Geometry check sheet. Reference: the model listing, model coordinates, mm. A direction names the side the tool comes from. Give positions to 0.01 mm unless a question says otherwise; leave off trailing zeros. Write each loop counter-clockwise with the first axis right and the second up, starting at its lowest first coordinate (ties: lowest second). Pieces come first, ordered by that corner, then holes. Notation, with made-up numbers: M 42,84.5 L 70,84.5 A24 cw 70,104.5 Z; hole C 0.5,9.5 d3. An arc over 180 degrees is marked long. One line per item, written item: value. Start each with the question number.
1. Release check for a two-part mould opening along Z. For faces 6 (the face through (64, 4, 2)), 7 (the face through (9.493, 68.474, 30.981)), 8 (the face through (61.86, 45.9, 19.74)) record: pulls with the +Z half, pulls with the -Z half, needs draft (parallel to the pull), parting line crosses it, or undercut.
2. Tool access check on faces 1 (the face through (-4, 82, 3)), 2 (the face through (67.43, 87.4, 19.27)), 3 (the face through (62.9, 5.1, 37)), 4 (the face through (68, 43, 19)), 5 (the face through (0, 26, 19)). Record the directions out of +Z, -Z, +X, -X, +Y, -Y that give a thin tool (end or side, any length) a straight path to the whole face; none if there is none.
3. Cross-section at B-B on x = 50. Record the cut outline in (y, z), then the cut area to 3 significant figures.
4. Cross-section at D-D on y = 10.5. Record the cut outline in (x, z), then the cut area to 3 significant figures.
5. Gauge pin test, flat ends, axial feed: pin 1 (3 mm diameter, centred on x = 64, y = 4.5, fed in from +Z); pin 2 (19 mm diameter, centred on y = 15, z = 13.5, fed in from -X); pin 3 (1.5 mm diameter, centred on y = 75, z = 13, fed in from -X). Record the tip position at first contact, or that the pin passes through.
6. Cross-section at A-A on y = 70. Count the separate pieces of the cut face and the enclosed holes in it, then the cut area to 3 significant figures.
7. Scan lines: line 1 (Z direction, x = 9.4, y = 70); line 2 (Y direction, x = 2.5, z = 17); line 3 (Y direction, x = 4, z = 22). Record each from-to range of solid material in increasing order.
from build123d import *

# Parameters (mm, degrees)
EXTRUDE_1_DEPTH     = 38
SHELL_1_T           = -2
SKETCH_9_W          = 20
SKETCH_9_H          = 34.8
EXTRUDE_3_DEPTH     = 6
SKETCH_9_3_W        = 20
SKETCH_9_3_H        = 1.2
EXTRUDE_4_DEPTH     = 38
FILLET_1_R          = 2
FILLET_2_R          = 4
FILLET_4_R          = 2
SKETCH_3_W          = 6
SKETCH_3_H          = 6
SKETCH_3_R          = 1.4
EXTRUDE_2_DEPTH     = 35
FILLET_3_R          = 3
SKETCH_2_R          = 3.75
SKETCH_2_R_2        = 1.6
CUT_EXTRUDE_1_DEPTH = 30
CHAMFER_1_SIZE      = 1
CUT_EXTRUDE_START   = -2
SKETCH_2_3_R        = 12.5
CUT_EXTRUDE_2_DEPTH = 5
CUT_EXTRUDE_START_2 = 1.2
CUT_EXTRUDE_4_DEPTH = 10
SKETCH_10_R         = 1.4
CUT_EXTRUDE_5_DEPTH = 8
SKETCH_11_W         = 56
SKETCH_11_H         = 6
SKETCH_11_R         = 1.4
EXTRUDE_5_DEPTH     = 6
SKETCH_11_2_R       = 1.4
CUT_EXTRUDE_6_DEPTH = 6


with BuildPart() as part:
    # 草图1 → 凸台-拉伸1 (new body)
    with BuildSketch(Plane.XY):
        Polygon((0, 0), (68, 0), (68, 88), (8, 88), (8, 52), (0, 52), align=None)
    extrude(amount=EXTRUDE_1_DEPTH)

    # 抽壳1
    shell_1_openings = [part.faces().sort_by_distance(p)[0] for p in [
        (35.516853933, 42.685393258, 38),
    ]]
    offset(amount=SHELL_1_T, openings=shell_1_openings, kind=Kind.INTERSECTION)

    # 草图9 → 凸台-拉伸3 (add)
    with BuildSketch(Plane.XY):
        with Locations((-2, 69.4)):
            Rectangle(SKETCH_9_W, SKETCH_9_H)
    extrude(amount=EXTRUDE_3_DEPTH)

    # 草图9<3> → 凸台-拉伸4 (add)
    with BuildSketch(Plane.XY):
        with Locations((-2, 87.4)):
            Rectangle(SKETCH_9_3_W, SKETCH_9_3_H)
    extrude(amount=EXTRUDE_4_DEPTH)

    # 圆角1
    fillet_1_edges = [part.edges().sort_by_distance(p)[0] for p in [
        (0, 0, 19),
        (8, 52, 22),
        (68, 88, 19),
        (68, 0, 19),
        (0, 52, 3),
        (8, 86.8, 22),
    ]]
    fillet(fillet_1_edges, radius=FILLET_1_R)

    # 圆角2
    fillet_2_edges = [part.edges().sort_by_distance(p)[0] for p in [
        (10, 50, 20),
        (-12, 52, 3),
    ]]
    fillet(fillet_2_edges, radius=FILLET_2_R)

    # 圆角4
    fillet_4_edges = [part.edges().sort_by_distance(p)[0] for p in [
        (0, 52, 22),
    ]]
    fillet(fillet_4_edges, radius=FILLET_4_R)

    # 草图3 → 凸台-拉伸2 (add)
    # profile 1 of 6: a face of its own
    with BuildSketch(Plane.XY.offset(2)):
        with Locations((64, 84)):
            Rectangle(SKETCH_3_W, SKETCH_3_H)
        with Locations((64, 84)):
            Circle(SKETCH_3_R, mode=Mode.SUBTRACT)
    # profile 2 of 6: a face of its own
    with BuildSketch(Plane.XY.offset(2)):
        with Locations((12, 84)):
            Rectangle(SKETCH_3_W, SKETCH_3_H)
        with Locations((12, 84)):
            Circle(SKETCH_3_R, mode=Mode.SUBTRACT)
    # profile 3 of 6: a face of its own
    with BuildSketch(Plane.XY.offset(2)):
        with Locations((64, 4)):
            Rectangle(SKETCH_3_W, SKETCH_3_H)
        with Locations((64, 4)):
            Circle(SKETCH_3_R, mode=Mode.SUBTRACT)
    # profile 4 of 6: a face of its own
    with BuildSketch(Plane.XY.offset(2)):
        with Locations((4, 48)):
            Rectangle(SKETCH_3_W, SKETCH_3_H)
        with Locations((4, 48)):
            Circle(SKETCH_3_R, mode=Mode.SUBTRACT)
    # profile 5 of 6: a face of its own
    with BuildSketch(Plane.XY.offset(2)):
        with Locations((4, 4)):
            Rectangle(SKETCH_3_W, SKETCH_3_H)
        with Locations((4, 4)):
            Circle(SKETCH_3_R, mode=Mode.SUBTRACT)
    # profile 6 of 6: a face of its own
    with BuildSketch(Plane.XY.offset(2)):
        with Locations((64, 48)):
            Rectangle(SKETCH_3_W, SKETCH_3_H)
        with Locations((64, 48)):
            Circle(SKETCH_3_R, mode=Mode.SUBTRACT)
    extrude(amount=EXTRUDE_2_DEPTH)

    # 圆角3
    fillet_3_edges = [part.edges().sort_by_distance(p)[0] for p in [
        (15, 81, 19.5),
        (61, 81, 19.5),
        (61, 7, 19.5),
        (7, 45, 19.5),
        (7, 7, 19.5),
        (61, 45, 19.5),
        (61, 51, 19.5),
    ]]
    fillet(fillet_3_edges, radius=FILLET_3_R - 0.0001)  # a hair under: the kernel refuses the full size

    # 草图2 → 切除-拉伸1 (cut)
    with BuildSketch(Plane.ZY.offset(-8)):
        with Locations(Location((22, 70, 0), (0, 0, 270))):
            Circle(SKETCH_2_R)
        with Locations(Location((30.5, 70, 0), (0, 0, 270))):
            Circle(SKETCH_2_R_2)
        with Locations(Location((13.5, 70, 0), (0, 0, 270))):
            Circle(SKETCH_2_R_2)
    extrude(amount=-CUT_EXTRUDE_1_DEPTH, mode=Mode.SUBTRACT)

    # 倒角1
    chamfer_1_edges = [part.edges().sort_by_distance(p)[0] for p in [
        (8, 71.6, 13.5),
        (8, 71.6, 30.5),
    ]]
    chamfer(chamfer_1_edges, length=CHAMFER_1_SIZE)

    # 草图2<3> → 切除-拉伸2 (cut)
    with BuildSketch(Plane.ZY.offset(-8).offset(CUT_EXTRUDE_START)):
        with Locations((22, 70)):
            Circle(SKETCH_2_3_R)
    extrude(amount=-CUT_EXTRUDE_2_DEPTH, mode=Mode.SUBTRACT)

    # 草图1<3> → 切除-拉伸4 (cut)
    with BuildSketch(Plane.XY.offset(CUT_EXTRUDE_START_2)):
        Polygon((8, 44), (8, 8), (60, 8), (60, 80), (16, 80), (16, 44), align=None)
    extrude(amount=CUT_EXTRUDE_4_DEPTH, mode=Mode.SUBTRACT)

    # 草图10 → 切除-拉伸5 (cut)
    with BuildSketch(Plane.ZY.offset(12)):
        with Locations(Location((3, 82, 0), (0, 0, 270))):
            Circle(SKETCH_10_R)
        with Locations(Location((3, 62, 0), (0, 0, 270))):
            Circle(SKETCH_10_R)
    extrude(amount=-CUT_EXTRUDE_5_DEPTH, mode=Mode.SUBTRACT)

    # 草图11 → 凸台-拉伸5 (add)
    with BuildSketch(Plane.XZ):
        with Locations((34, 3)):
            Rectangle(SKETCH_11_W, SKETCH_11_H)
        with Locations((10, 3)):
            Circle(SKETCH_11_R, mode=Mode.SUBTRACT)
        with Locations((34, 3)):
            Circle(SKETCH_11_R, mode=Mode.SUBTRACT)
        with Locations((58, 3)):
            Circle(SKETCH_11_R, mode=Mode.SUBTRACT)
    extrude(amount=-EXTRUDE_5_DEPTH)

    # 草图11<2> → 切除-拉伸6 (cut)
    with BuildSketch(Plane.XZ):
        with Locations(Location((10, 3, 0), (0, 0, 270))):
            Circle(SKETCH_11_2_R)
        with Locations(Location((58, 3, 0), (0, 0, 270))):
            Circle(SKETCH_11_2_R)
        with Locations(Location((34, 3, 0), (0, 0, 270))):
            Circle(SKETCH_11_2_R)
    extrude(amount=-CUT_EXTRUDE_6_DEPTH, mode=Mode.SUBTRACT)


solid = part.part
Report:
1. face 6: pulls with the +Z half
1. face 7: undercut
1. face 8: needs draft
2. face 1: -X
2. face 2: +Z, -Z, +X, +Y
2. face 3: +Z
2. face 4: +Z, -Z, +X, +Y, -Y
2. face 5: +Z, -Z, -X, -Y
3. outline: M 0,0 L 88,0 L 88,38 L 86,38 L 86,2 L 80,2 L 80,1.2 L 8,1.2 L 8,2 L 6,2 L 6,6 L 2,6 L 2,38 L 0,38 Z
3. area: 278 mm^2
4. outline: M 0,0 L 68,0 L 68,38 L 66,38 L 66,2 L 60,2 L 60,1.2 L 8,1.2 L 8,2 L 2,2 L 2,38 L 0,38 Z
4. area: 238 mm^2
5. pin 1: stops at z = 37
5. pin 2: stops at x = 0
5. pin 3: stops at x = 8
6. separate pieces: 4
6. enclosed holes: 0
6. area: 319 mm^2
7. line 1: z = 0 to 11.9, 15.1 to 18.25, 25.75 to 28.9, 32.1 to 38
7. line 2: y = 0 to 7, 45 to 52, 86.8 to 88
7. line 3: y = 0 to 2.6, 5.4 to 7, 45 to 46.6, 49.4 to 52, 86.8 to 88
